For this review, take the finished solid that the model builds, in its own axes (mm). Face numbers are marked on the shaded views. A direction names the side the tool comes from. Give positions to 0.01 mm unless a question says otherwise; leave off trailing zeros. Order: outer loops, then holes, each group sorted by start corner. A loop starts at its lowest first (then second) coordinate and runs counter-clockwise, first axis right, second up.
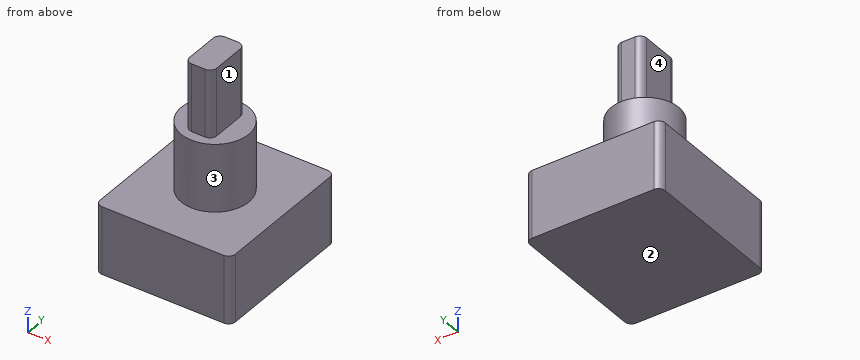
Autodesk Fusion 360 part; units mm, degrees
sketch "Sketch1" plane through (0, 0, 0) normal (0, 0, 1) x (1, 0, 0)
  line L0 (5, 5.5) -> (-5, 5.5)
  line L1 (-5, 5.5) -> (-5, -5.5)
  line L2 (-5, -5.5) -> (5, -5.5)
  line L3 (5, -5.5) -> (5, 5.5)
  line L4 (5, 5.5) -> (-5, -5.5) construction
  line L5 (-5, 5.5) -> (5, -5.5) construction
  dimension "d1" = 10
  dimension "d2" = 11
extrude "Extrude1" add sketch "Sketch1" along normal blind 5
sketch "Sketch2" plane through (0, 0, 5) normal (0, 0, 1) x (-1, 0, 0)
  line L0 (-5, 5.5) -> (-5, -5.5)
  line L1 (-5, -5.5) -> (5, -5.5)
  line L2 (5, -5.5) -> (5, 5.5)
  line L3 (5, 5.5) -> (-5, 5.5)
  circle A0 centre (0, 0) radius 2.5
  dimension "d5" = 5
extrude "Extrude2" add sketch "Sketch2" along normal blind 10 contours A0
sketch "Sketch3" plane through (0, 0, 15) normal (0, 0, 1) x (-1, 0, 0)
  circle A0 centre (0, 0) radius 2.5
  line L0 (-1, -1.75) -> (1, -1.75)
  line L1 (1, -1.75) -> (1, 1.75)
  line L2 (1, 1.75) -> (-1, 1.75)
  line L3 (-1, 1.75) -> (-1, -1.75)
  line L4 (-1, -1.75) -> (1, 1.75) construction
  line L5 (1, -1.75) -> (-1, 1.75) construction
  dimension "d8" = 2
  dimension "d9" = 3.5
extrude "Extrude3" cut sketch "Sketch3" against normal blind 5
fillet "Fillet1" radius 0.5 4 edges at (-1, -1.75, 12.5) (1, -1.75, 12.5) (-1, 1.75, 12.5) (1, 1.75, 12.5)
fillet "Fillet2" radius 0.5 4 edges at (-5, 5.5, 2.5) (5, 5.5, 2.5) (-5, -5.5, 2.5) (5, -5.5, 2.5)
1) We need section A-A on x = 0. Give the boundary of the cut face in (y, z).
Answer sheet:
outline: (-5.5, 0) - (5.5, 0) - (5.5, 5) - (2.5, 5) - (2.5, 10) - (1.75, 10) - (1.75, 15) - (-1.75, 15) - (-1.75, 10) - (-2.5, 10) - (-2.5, 5) - (-5.5, 5) - close
2) We need section B-B on y = 0. Give the boundary of the cut face in (x, z), then the cut area to 3 significant figures.
Answer sheet:
outline: (-5, 0) - (5, 0) - (5, 5) - (2.5, 5) - (2.5, 10) - (1, 10) - (1, 15) - (-1, 15) - (-1, 10) - (-2.5, 10) - (-2.5, 5) - (-5, 5) - close
area: 85.0 mm2
3) To check wall thickness, follow line 1 (Z direction, x = -3, y = 1.5); line 2 (Z direction, x = 0.75, y = 2.25); line 3 (Y direction, x = 0.25, z = 14). State the ranges of each line that lie inside material, in increasing order.
Answer sheet:
line 1: z = 0 to 5
line 2: z = 0 to 10
line 3: y = -1.75 to 1.75
4) We need section D-D on x = 1.5. Give the boundary of the cut face in (y, z), then the cut area to 3 significant figures.
Answer sheet:
outline: (-5.5, 0) - (5.5, 0) - (5.5, 5) - (2, 5) - (2, 10) - (-2, 10) - (-2, 5) - (-5.5, 5) - close
area: 75.0 mm2
5) We need section C-C on z = 7.5. Give the boundary of the cut face in (x, y), then the cut area to 3 significant figures.
Answer sheet:
outline: circle Ø5 at (0, 0)
area: 19.6 mm2
6) Clearance check with flat-ended pins moving along their axes: pin 1 (4 mm diameter, centred on x = 2.5, z = 12, fed in from +Y); pin 2 (1.2 mm diameter, centred on y = 0, z = 13, fed in from -X); pin 3 (1.2 mm diameter, centred on y = 0, z = 13, fed in from +X). State where each tip first meets the part, or that it passes through.
Answer sheet:
pin 1: stops at y = 1.75
pin 2: stops at x = -1
pin 3: stops at x = 1
7) Tool access review of the marked faces 1, 2, 3 and 4: name each direction out of +Z, -Z, +X, -X, +Y, -Y from which nothing blocks a thin tool from reaching the whole face with its end or side.
Answer sheet:
face 1: +Z, +X, +Y, -Y
face 2: -Z, +X, -X, +Y, -Y
face 3: +Z
face 4: +Z, -X, +Y, -Y
